Part print with two shaded views. Sizes in mm from the minimum x, y, z corner. Round coordinates to 2 decimals unless told otherwise and drop trailing zeros. Write each loop counter-clockwise with the first axis right and the second up, starting at its lowest first coordinate (ties: lowest second). Pieces come first, ordered by that corner, then holes. Notation, with made-up numbers: (16, 28) -> (75, 28) arc R20 cw to (75, 51) -> close; hole circle Ø2 at (62.5, -21.75). An arc over 180 degrees is marked (long way). Answer in a Markdown table with one row per item. Add a question column.
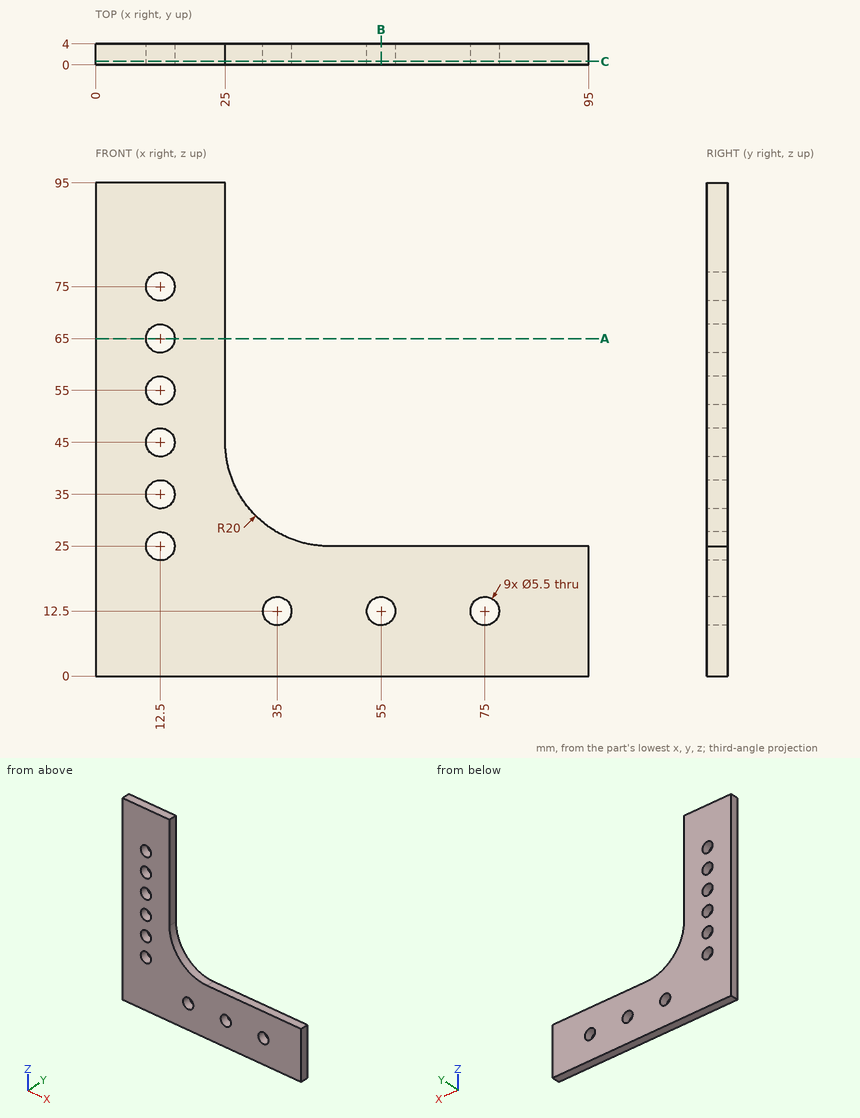
Item 1: Saw through at C-C on y = 0.65. Count the separate pieces of the cut face and the enclosed holes in it, then the cut area to 3 significant figures.
Item 2: Saw through at A-A on z = 65. Give the cut face in (x, y).
Item 3: Saw through at B-B on x = 55. Give the cut face in (y, z).
Item 4: Pin check, flat tips, straight feed: pin 1 (2 mm diameter, centred on x = 79.5, y = 2.5, fed in from +Z); pin 2 (2 mm diameter, centred on x = 37.5, y = 2, fed in from +Z). Stop position of each tip, or through.
Item 5: Drill centre lines: probe 1 along Z at (x, y) = (49, 1.2); probe 2 along X at (y, z) = (3.35, 77.5). Where is each one in solid material? Low to high.
Recorded:
| question | item | result |
|---|---|---|
| 1 | separate pieces | 1 |
| 1 | enclosed holes | 9 |
| 1 | area | 4,000 mm2 |
| 2 | outline | (0, 0) -> (9.75, 0) -> (9.75, 4) -> (0, 4) -> close; (15.25, 0) -> (25, 0) -> (25, 4) -> (15.25, 4) -> close |
| 3 | outline | (0, 0) -> (4, 0) -> (4, 9.75) -> (0, 9.75) -> close; (0, 15.25) -> (4, 15.25) -> (4, 25) -> (0, 25) -> close |
| 4 | pin 1 | z = 25 |
| 4 | pin 2 | z = 26.9 |
| 5 | probe 1 | 0 to 25 |
| 5 | probe 2 | 0 to 11.35, 13.65 to 25 |
